Verification items for the finished model (mm, model axes). A direction names the side the tool comes from. Give positions to 0.01 mm unless a question says otherwise; leave off trailing zeros. Write each loop counter-clockwise with the first axis right and the second up, starting at its lowest first coordinate (ties: lowest second). Pieces come first, ordered by that corner, then holes. Notation, with made-up numbers: (-4.5, 33) -> (4.5, 33) arc R25 ccw to (4.5, 70) -> close; hole circle Ø5 at (-7.5, -37). An arc over 180 degrees is marked (long way). Use CSV: the item, a comma, the result in double quotes. Start each with the question number.
```python
from build123d import *

# Parameters (mm, degrees)
F0_W          = 150
F0_H          = 50
F1_DEPTH      = 148.9
F2_T          = -3
F3_W          = 149.098023
F3_H          = 8.212631
F4_DEPTH      = 98.5
F4_DEPTH_BACK = 98.4


with BuildPart() as f1:
    # F0 (on Front) → F1 (new body)
    with BuildSketch(Plane.XZ):
        Rectangle(F0_W, F0_H)
    extrude(amount=F1_DEPTH)

    # F2
    f2_openings = [f1.faces().sort_by_distance(p)[0] for p in [
        (0, -148.9, 0),
    ]]
    offset(amount=F2_T, openings=f2_openings)

    # F3 (on Right) → F4 (cut, two sides)
    with BuildSketch(Plane.YZ) as f4_sk:
        with Locations((-82.449026, 0.456257)):
            Rectangle(F3_W, F3_H)
    extrude(amount=F4_DEPTH, mode=Mode.SUBTRACT)
    extrude(f4_sk.sketch, amount=-F4_DEPTH_BACK, mode=Mode.SUBTRACT)


solid = f1.part
```
(1) Go/stop test with flat-tipped pins: pin 1 (0.9 mm diameter, centred on x = -74, z = -1.5, fed in from -Y); pin 2 (10 mm diameter, centred on x = 23, z = 1.5, fed in from -Y). Record where each tip stops, or that it passes through.
(2) Section check C-C on z = 7.5. Record the cut outline in (x, y), then the cut area to 3 significant figures.
(3) Set-up check for faces 1 (the face through (-1, -3, 0)), 2 (the face through (75, -73, 5)): record each of +Z, -Z, +X, -X, +Y, -Y from which the full face is reachable in a straight line by a thin tool's end or side.
(4) Draft check along X on faces 3 (the face through (-75, -73, 5)), 4 (the face through (-1, -73, -25)), 5 (the face through (-1, -75, 22)). Enter one of: released by +X, released by -X, zero draft, split by the parting line, or undercut.
(5) Section check B-B on x = -30. Record the cut outline in (y, z), then the cut area to 3 significant figures.
(6) Thickness scan on line 1 (Z direction, x = 38.5, y = -40.5); line 2 (X direction, y = -42.5, z = 14.5); line 3 (Y direction, x = -2.5, z = 20.5). Record the ranges inside material, lowest first. Write a range as from..to.
(7) Section check A-A on y = -49.5. Record the cut outline in (x, z), then the cut area to 3 significant figures.
Data:
1,pin 1,"stops at y = -7.9"
1,pin 2,"stops at y = -3"
2,outline,"(-75, -148.9) -> (-72, -148.9) -> (-72, -3) -> (72, -3) -> (72, -148.9) -> (75, -148.9) -> (75, 0) -> (-75, 0) -> close"
2,area,"1,330 mm2"
3,face 1,"-Y"
3,face 2,"+Z, -Z, +X, +Y, -Y"
4,face 3,"released by -X"
4,face 4,"zero draft"
4,face 5,"undercut"
5,outline,"(-148.9, -25) -> (0, -25) -> (0, 25) -> (-148.9, 25) -> (-148.9, 22) -> (-3, 22) -> (-3, -22) -> (-148.9, -22) -> close"
5,area,"1,030 mm2"
6,line 1,"z = -25..-22, 22..25"
6,line 2,"x = -75..-72, 72..75"
6,line 3,"y = -3..0"
7,outline,"(-75, -25) -> (75, -25) -> (75, -3.65) -> (72, -3.65) -> (72, -22) -> (-72, -22) -> (-72, -3.65) -> (-75, -3.65) -> close; (-75, 4.56) -> (-72, 4.56) -> (-72, 22) -> (72, 22) -> (72, 4.56) -> (75, 4.56) -> (75, 25) -> (-75, 25) -> close"
7,area,"1,110 mm2"
